Design review of the part built by this model. Coordinates are the model's own, in mm. Coordinates: 2 decimals unless noted, no trailing zeros. Loops run counter-clockwise (first coordinate to the right, second up) from the corner with the lowest first, then second, coordinate; pieces in that order, holes last. Notation, with made-up numbers: M 30.5,33.25 L 85.5,33.25 A23 ccw 85.5,49.25 Z; hole C 88,64.5 d7. An arc over 180 degrees is marked long. Write item = value, one per line. Start each with the question number.
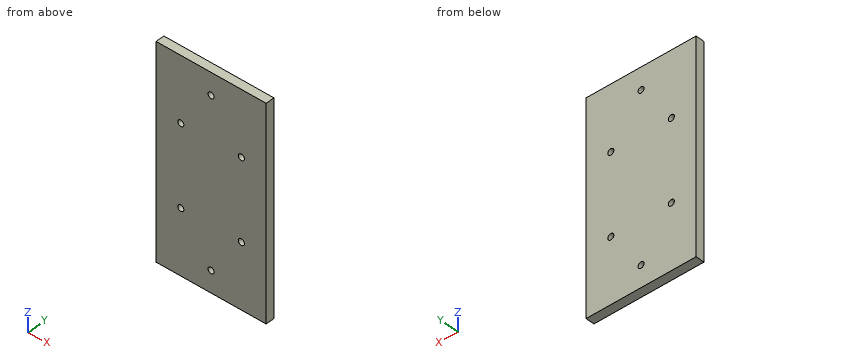
Autodesk Fusion 360 part; units mm, degrees
sketch "Sketch1" plane through (0, 0, 0) normal (0, 1, 0) x (1, 0, 0)
  line L0 (-27.26, -52) -> (-27.26, 52)
  line L1 (-27.26, 52) -> (27.26, 52)
  line L2 (27.26, 52) -> (27.26, -52)
  line L3 (0, 80) -> (0, -60) construction
  line L4 (-60, 0) -> (45.848, 0) construction
  line L5 (-15, 52) -> (-15, 35.15) construction
  line L6 (-15, 35.15) -> (15, 35.15) construction
  line L7 (15, 35.15) -> (15, 52) construction
  circle A0 centre (0, 41.325) radius 6.175
  line L8 (-15, 52) -> (-15, 20) construction
  line L9 (-15, 20) -> (15, 20) construction
  line L10 (15, 20) -> (15, 52) construction
  line L11 (-15, 20) -> (-15, -20) construction
  line L12 (-15, -20) -> (15, -20) construction
  line L13 (15, -20) -> (15, 20) construction
  line L14 (27.26, -52) -> (-27.26, -52)
  line L15 (15, -52) -> (15, -35) construction
  line L16 (15, -35) -> (-15, -35) construction
  line L17 (-15, -35) -> (-15, -52) construction
  line L18 (-15, -20) -> (-15, -35) construction
  line L19 (15, -20) -> (15, -35) construction
  circle A1 centre (0, -41.175) radius 6.175
  dimension "d2" = 54.52
  dimension "d6" = 16.85
  dimension "d7" = 12.35
  dimension "d9" = 32
  dimension "d10" = 40
  dimension "d12" = 104
  dimension "d16" = 17
  dimension "d17" = 12.35
extrude "Extrude1" add sketch "Sketch1" against normal blind 4.3 contours L0 L1 L2 L14 | A0 | A1
sketch "Sketch2" plane through (0, 0, 0) normal (0, 1, 0) x (1, 0, 0)
  circle A0 centre (-15, -20) radius 1.5
  circle A1 centre (15, -20) radius 1.5
  circle A2 centre (-15, 20) radius 1.5
  circle A3 centre (15, 20) radius 1.5
  circle A4 centre (0, 41.325) radius 1.5
  circle A5 centre (0, -41.175) radius 1.5
  dimension "d20" = 3
  dimension "d21" = 3
  dimension "d22" = 3
  dimension "d23" = 3
  dimension "d24" = 3
  dimension "d25" = 3
extrude "Extrude2" cut sketch "Sketch2" against normal up to surface (4.3 mm away)
(1) Take a section at A-A (x = -15). State the section outline as (y, z) points, plus the area to 3 significant figures.
(2) To check wall thickness, follow L1, parallel to X at y = -2.6, z = -20; L2, parallel to Z at x = -15, y = -2.75; L3, parallel to Z at x = 0, y = -2.55 (3 decimals). State the ranges of each line that lie inside material, in increasing order.
(3) Take a section at B-B (z = 20). State the section outline as (x, y) points.
(4) Insertion check: pin 1 (1.8 mm diameter, centred on x = -15, z = -20, fed in from -Y); pin 2 (3.5 mm diameter, centred on x = -15, z = 20, fed in from -Y). Each pin has a flat end and moves straight along its axis. Give the tip position at first contact, or say it passes through.
Results list:
q1.outline = M -4.3,-52 L 0,-52 L 0,-21.5 L -4.3,-21.5 Z; M -4.3,-18.5 L 0,-18.5 L 0,18.5 L -4.3,18.5 Z; M -4.3,21.5 L 0,21.5 L 0,52 L -4.3,52 Z
q1.area = 421 mm^2
q2.L1 = -27.26 to -16.5, -13.5 to 13.5, 16.5 to 27.26
q2.L2 = -52 to -21.5, -18.5 to 18.5, 21.5 to 52
q2.L3 = -52 to -42.825, -39.825 to 39.675, 42.675 to 52
q3.outline = M -27.26,-4.3 L -16.5,-4.3 L -16.5,0 L -27.26,0 Z; M -13.5,-4.3 L 13.5,-4.3 L 13.5,0 L -13.5,0 Z; M 16.5,-4.3 L 27.26,-4.3 L 27.26,0 L 16.5,0 Z
q4.pin_1 = through
q4.pin_2 = -4.3
